Can you work these out from the model? Positions are in its coordinate system, mm. Face numbers are marked on the shaded views. Give positions to 0.01 mm unless a question says otherwise; leave off trailing zeros. Loops run counter-clockwise (first coordinate to the right, second up) from the corner with the lowest first, then second, coordinate; pieces in that order, holes last. Notation, with made-up numbers: (21, 21.25) - (37, 21.25) arc R34 cw to (37, 60.25) - close; hole circle Ø1 at (-33.75, 1.5). An arc over 180 degrees is marked (long way). Write item = value, one per line.
from build123d import *

# Parameters (mm, degrees)
F0_W      = 45
F0_H      = 110
F0_H_2    = 15
F0_W_2    = 20
F0_H_3    = 100
F0_W_3    = 55
F1_DEPTH  = 3
F2_R      = 5
F3_R      = 2.99999
F5_D      = 2
F6_W      = 70
F6_H      = 82
F7_DEPTH  = 1.5
F8_W      = 46.3650951658
F8_H      = 25.5117665604
F9_DEPTH  = 8
F11_D     = 2
F11_DEPTH = 6
F11_TIP   = 0.600860619


# Not quite as in the source:
# - a fillet or chamfer is up to 0.001 mm smaller than in the source, because OpenCascade refuses the exact size


with BuildPart() as f1:
    # F0 (on Top) → F1 (new body)
    with BuildSketch(Plane.XY):
        with Locations((-49.1538274859, -4.7530609369)):
            Rectangle(F0_W, F0_H)
        Polygon((43.3461725141, 50.2469390631), (-26.6538274859, 50.2469390631), (-26.6538274859, -59.7530609369), (28.3461725141, -59.7530609369), (46.3587938504, -49.7530609369), (46.3587938504, 50.2469390631), align=None)
        with Locations((-49.1538274859, -67.2530609369)):
            Rectangle(F0_W, F0_H_2)
        with Locations((56.3587938504, 0.2469390631)):
            Rectangle(F0_W_2, F0_H_3)
        with Locations((0.8461725141, -67.2530609369)):
            Rectangle(F0_W_3, F0_H_2)
        Polygon((-26.6538274859, 80.2469390631), (-26.6538274859, 50.2469390631), (43.3461725141, 50.2469390631), (43.3461725141, 70.4786608508), (43.3461725141, 80.2469390631), align=None)
        Polygon((43.3461725141, 70.4786608508), (43.3461725141, 50.2469390631), (46.3587938504, 50.2469390631), (66.3587938504, 50.2469390631), (66.3587938504, 70.4786608508), align=None)
        Polygon((43.3461725141, 80.2469390631), (43.3461725141, 70.4786608508), (66.3587938504, 70.4786608508), align=None)
    extrude(amount=F1_DEPTH)

    # F2
    f2_edges = [f1.edges().sort_by_distance(p)[0] for p in [
        (-26.653827, 50.246939, 1.5),
    ]]
    fillet(f2_edges, radius=F2_R)

    # F3 (radius 3 in the source; OpenCascade refuses exactly that, so slightly less here)
    f3_edges = [f1.edges().sort_by_distance(p)[0] for p in [
        (-26.653827, 67.746939, 0),
        (-28.118294, 51.711405, 0),
        (8.346173, 80.246939, 0),
        (-51.653827, 50.246939, 0),
        (54.852483, 75.3628, 0),
        (-71.653827, -12.253061, 0),
        (66.358794, 10.3628, 0),
        (-21.653827, -74.753061, 0),
        (56.358794, -49.753061, 0),
        (28.346173, -67.253061, 0),
        (37.352483, -54.753061, 0),
    ]]
    fillet(f3_edges, radius=F3_R)

    # F5 (through all)
    with Locations(Plane.XY.offset(3)):
        with Locations((-65.6538274859, 17.2469390631), (-64.6538274859, -68.7530609369), (23.3461725141, -47.7530609369), (53.3587938504, -28.7530609369), (53.3587938504, 2.9659790631), (61.3461725141, 50.2469390631), (33.3461725141, 74.2469390631), (-28.6538274859, 46.2469390631)):
            Hole(F5_D / 2)

    # F6 (on face) → F7 (cut)
    with BuildSketch(Plane.XY.offset(3)):
        with Locations((-24.6538274859, -0.7530609369)):
            Rectangle(F6_W, F6_H)
        Polygon((-61.6538274859, -41.7530609369), (-61.6538274859, -71.7530609369), (12.3461725141, -71.7530609369), (12.3461725141, -41.7530609369), (10.3461725141, -41.7530609369), (-59.6538274859, -41.7530609369), align=None)
    extrude(amount=-F7_DEPTH, mode=Mode.SUBTRACT)

    # F8 (on face) → F9 (join)
    with BuildSketch(Plane.XY.offset(3)):
        Polygon((-15.3889879584, 70.8764791489), (-15.3889879584, 40.2469390631), (10.3461725141, 40.2469390631), (56.7112676799, 40.2469390631), (56.7112676799, 70.8764791489), align=None)
        with Locations((33.528720097, 27.4910557829)):
            Rectangle(F8_W, F8_H)
    extrude(amount=F9_DEPTH)

    # F11
    with Locations(Plane.XY.offset(11)):
        with Locations((-8.1770029031, 59.1886730194), (42.8229970969, 65.1886730194), (42.8229970969, 18.1886730194)):
            Hole(F11_D / 2, depth=F11_DEPTH)
            with Locations((0, 0, -(F11_DEPTH + F11_TIP / 2))):  # 118° drill point
                Cone(0, F11_D / 2, F11_TIP, mode=Mode.SUBTRACT)


solid = f1.part
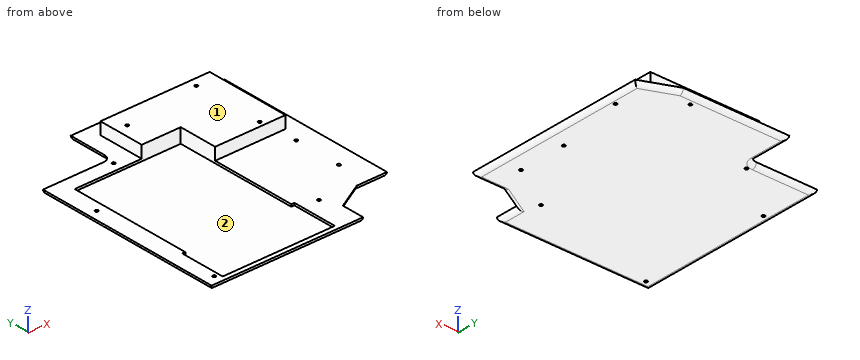
Q1. I need wall thicknesses on L1, parallel to Y at x = -14.5, z = 2.5; L2, parallel to Z at x = -55, y = -28; L3, parallel to Z at x = 34, y = -3. Which ranges of each line are inside material? Lowest first, please.
Output:
L1 = -74.71 to -71.75, 40.25 to 80.2
L2 = 0 to 1.5
L3 = 0 to 3
Q2. We'd pull the mould along X, two halves only. Please class the marked faces 1 and 2: released by +X, released by -X, zero draft, split by the parting line, or undercut.
Output:
face_1 = zero draft
face_2 = undercut
Q3. For pin 1 (2.5 mm diameter, centred on x = 61.35, y = 50.25, fed in from +Z); pin 2 (2.5 mm diameter, centred on y = 63, z = 6.5, fed in from -X); pin 3 (1.2 mm diameter, centred on y = 17.5, z = 2, fed in from +X); pin 4 (3 mm diameter, centred on y = -11, z = 6, fed in from -X), each with a flat end and sliding along its axis, tell me the tip position at first contact or that it passes through.
Output:
pin_1 = 3
pin_2 = -15.39
pin_3 = 66.33
pin_4 = through
Q4. Imagine slicing it at B-B, the plane z = 7. Write out the boundary of the cut face in (x, y).
Output:
outline = (-15.39, 40.25) - (10.35, 40.25) - (10.35, 14.74) - (56.71, 14.74) - (56.71, 70.88) - (-15.39, 70.88) - close; hole circle Ø2 at (-8.18, 59.19); hole circle Ø2 at (42.82, 18.19); hole circle Ø2 at (42.82, 65.19)
